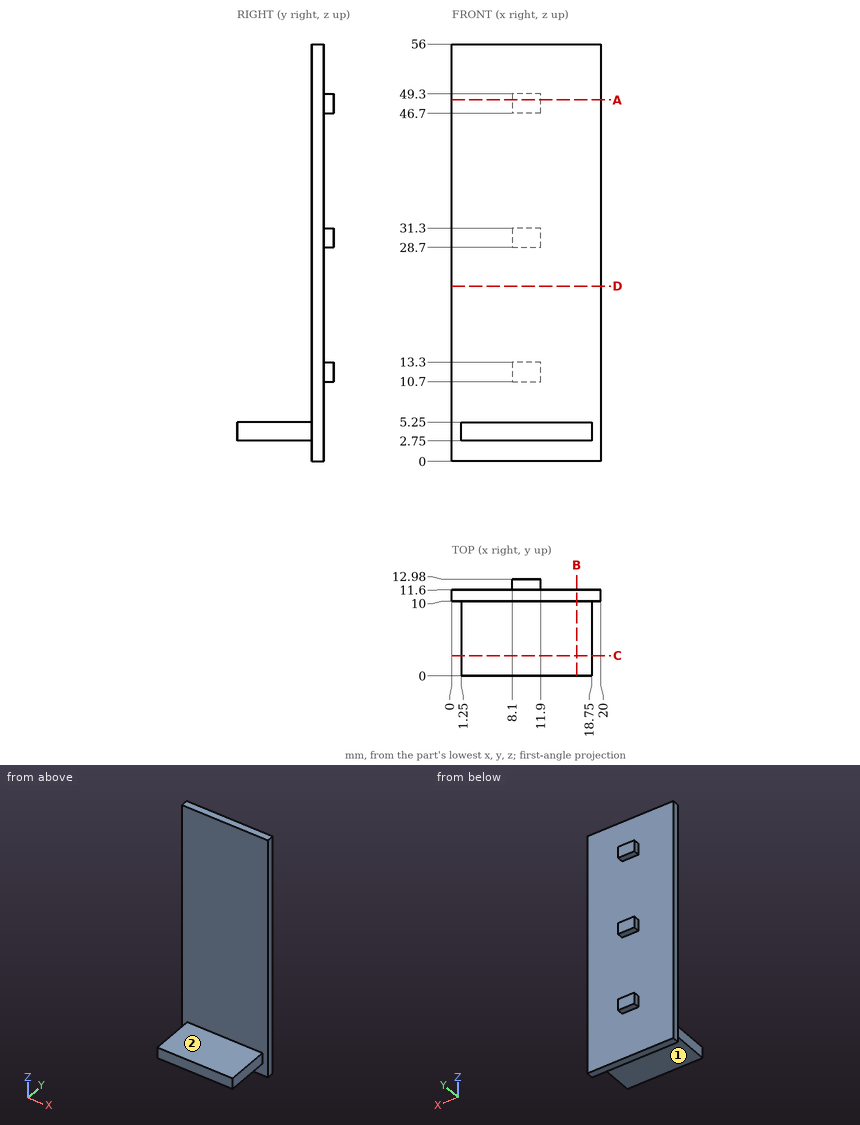
Input: dimensioned drawing with shaded views. Units: mm. Origin: part minimum x, y, z. A direction names the side the tool comes from. Give positions to 0.01 mm unless a question says otherwise; leave off trailing zeros. Order: outer loops, then holes, each group sorted by start corner. A loop starts at its lowest first (then second) coordinate and runs counter-clockwise, first axis right, second up. Notation, with made-up numbers: (61, 9.25) -> (97, 9.25) arc R33 ccw to (97, 41.25) -> close; hole circle Ø8 at (47, 47). An arc over 180 degrees is marked (long way). Write item = value, one per line.
Item 1: Section query D-D (z = 23.5). Output: boundary loops of the cut face in (x, y).
Check result:
outline = (0, 10) -> (20, 10) -> (20, 11.6) -> (0, 11.6) -> close
Item 2: Ray query, probe 1 along Z at (x, y) = (11, 8); probe 2 along Y at (x, z) = (18.75, 28.5); probe 3 along X at (y, z) = (5, 3). Return the intervals inside material, ascending.
Check result:
probe_1 = 2.75 to 5.25
probe_2 = 10 to 11.6
probe_3 = 1.25 to 18.75
Item 3: Contact query for flat-ended pins moving along their axis: pin 1 (4 mm diameter, centred on x = 15, z = 22.5, fed in from +Y); pin 2 (0.7 mm diameter, centred on x = 10.5, y = 12.5, fed in from +Z); pin 3 (0.7 mm diameter, centred on y = 12, z = 30.5, fed in from +X). Output: stop coordinate, or through.
Check result:
pin_1 = 11.6
pin_2 = 49.3
pin_3 = 11.9
Item 4: Set-up query: the marked faces 1 and 2. Return all of +Z, -Z, +X, -X, +Y, -Y with unobstructed straight access to the full face (end or side cutting, diameter ignored); none if empty.
Check result:
face_1 = -Z, +X, -X, -Y
face_2 = +Z, +X, -X, -Y
Item 5: Section query B-B (x = 16.75). Output: boundary loops of the cut face in (y, z).
Check result:
outline = (0, 2.75) -> (10, 2.75) -> (10, 0) -> (11.6, 0) -> (11.6, 56) -> (10, 56) -> (10, 5.25) -> (0, 5.25) -> close
Item 6: Section query C-C (y = 2.75). Output: boundary loops of the cut face in (x, z), then the cut area to 4 significant figures.
Check result:
outline = (1.25, 2.75) -> (18.75, 2.75) -> (18.75, 5.25) -> (1.25, 5.25) -> close
area = 43.75 mm²
Item 7: Section query A-A (z = 48.5). Output: boundary loops of the cut face in (x, y), then the cut area to 3 significant figures.
Check result:
outline = (0, 10) -> (20, 10) -> (20, 11.6) -> (11.9, 11.6) -> (11.9, 12.98) -> (8.1, 12.98) -> (8.1, 11.6) -> (0, 11.6) -> close
area = 37.2 mm²
